```python
from build123d import *

# Parameters (mm, degrees)
SKETCH1_W           = 7.95
SKETCH1_H           = 6.1
BOSS_EXTRUDE1_DEPTH = 7.95
CUT_EXTRUDE1_DEPTH  = 17.7
SKETCH3_W           = 4.95
SKETCH3_H           = 4.95
CUT_EXTRUDE2_DEPTH  = 1.7


with BuildPart() as part:
    # Sketch1 → Boss-Extrude1 (new body)
    with BuildSketch(Plane(origin=(0, 0, 0), x_dir=(0, 0, -1), z_dir=(1, 0, 0))):
        with Locations((3.975, -3.05)):
            Rectangle(SKETCH1_W, SKETCH1_H)
    extrude(amount=-BOSS_EXTRUDE1_DEPTH)

    # Sketch2 → Cut-Extrude1 (cut)
    with BuildSketch(Plane(origin=(0, 0, 0), x_dir=(0, 0, -1), z_dir=(1, 0, 0))):
        Polygon((7.95, 0), (0, -5.1), (0, 0), align=None)
    extrude(amount=-CUT_EXTRUDE1_DEPTH, mode=Mode.SUBTRACT)

    # Sketch3 → Cut-Extrude2 (cut)
    with BuildSketch(Plane.XZ.offset(6.1)):
        with Locations((-3.975, -3.975)):
            Rectangle(SKETCH3_W, SKETCH3_H)
    extrude(amount=-CUT_EXTRUDE2_DEPTH, mode=Mode.SUBTRACT)


solid = part.part
```
The listing builds one solid part. Answer for the finished solid, in the listing's coordinates (mm). A direction names the side the tool comes from. Round coordinates to 2 decimals unless told otherwise and drop trailing zeros. Write each loop counter-clockwise with the first axis right and the second up, starting at its lowest first coordinate (ties: lowest second). Pieces come first, ordered by that corner, then holes. Notation, with made-up numbers: (-5.5, 4.25) -> (40.5, 4.25) arc R21 ccw to (40.5, 27.25) -> close; hole circle Ø2 at (43, 22.5). An arc over 180 degrees is marked (long way). Answer as a JSON object with one key per item and string values. Group by question number.
Q1. Section C-C (z = -3) is taken. Write down the section's boundary in (x, y).
Q2. Determine the mould class of faces 3 (the face through (0, -4, -5)), 4 (the face through (-4, -4.4, -4)), 5 (the face through (-4, -3, -7.95)) for opening direction X: pulls with the +X half, pulls with the -X half, needs draft (parallel to the pull), parting line crosses it, or undercut.
Q3. This flat-tipped pin is pushed along its axis until it touches: pin 1 Ø2 at (x, y) = (-5.5, -4) entering from +Z. Where does it stop, or does it pass through?
Q4. Section D-D (y = -1) is taken. Write down the section's boundary in (x, z).
Q5. Which of the six approach directions +Z, -Z, +X, -X, +Y, -Y give full straight-line access (tool end or side, diameter ignored) to faces 1 (the face through (-4, -5, -1.5)), 2 (the face through (-3.9, -5.6, 0))?
Q6. Straight lines are drawn through the part: line 1 along X through (y, z) = (-5, -5.25); line 2 along Z through (x, y) = (-6, -5); line 3 along Y through (x, z) = (-3, -1.75). For each, find the intervals that lie inside material, in ascending order.
Q7. Section B-B (x = -5.5) is taken. Write down the section's boundary in (y, z).
Q8. Section A-A (y = -5.25) is taken. Write down the section's boundary in (x, z), plus the area to 3 significant figures.
Check values:
{
 "1": {"outline": "(-7.95, -6.1) -> (-6.45, -6.1) -> (-6.45, -4.4) -> (-1.5, -4.4) -> (-1.5, -6.1) -> (0, -6.1) -> (0, -3.18) -> (-7.95, -3.18) -> close"},
 "2": {"face 3": "pulls with the +X half", "face 4": "undercut", "face 5": "needs draft"},
 "3": {"pin 1": "z = -0.16"},
 "4": {"outline": "(-7.95, -7.95) -> (0, -7.95) -> (0, -6.39) -> (-7.95, -6.39) -> close"},
 "5": {"face 1": "-Y", "face 2": "+Z, +X, -X, +Y, -Y"},
 "6": {"line 1": "-7.95 to -6.45, -1.5 to 0", "line 2": "-7.95 to -6.45, -1.5 to -0.16", "line 3": "-4.4 to -3.98"},
 "7": {"outline": "(-6.1, -7.95) -> (0, -7.95) -> (-5.1, 0) -> (-6.1, 0) -> (-6.1, -1.5) -> (-4.4, -1.5) -> (-4.4, -6.45) -> (-6.1, -6.45) -> close"},
 "8": {"outline": "(-7.95, -7.95) -> (0, -7.95) -> (0, 0) -> (-7.95, 0) -> close; hole (-6.45, -6.45) -> (-1.5, -6.45) -> (-1.5, -1.5) -> (-6.45, -1.5) -> close", "area": "38.7 mm^2"}
}
